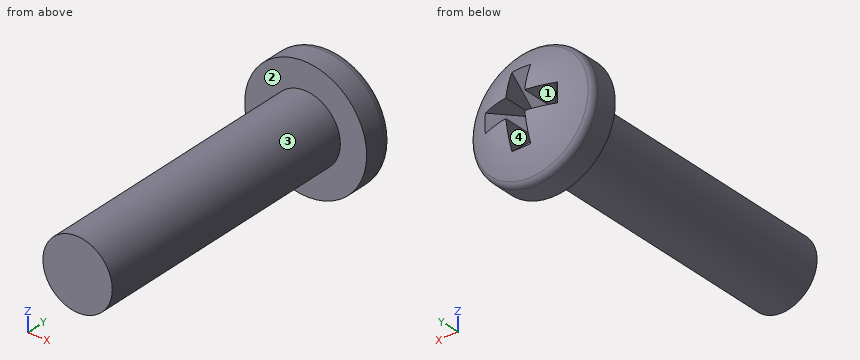
from build123d import *

# Parameters (mm, degrees)
SKETCH2_W          = 1.5875
SKETCH2_H          = 12.7
CUT_EXTRUDE1_DEPTH = 0.4318
CUT_EXTRUDE2_DEPTH = 0.4318


with BuildPart() as part:
    # Sketch1 → Base-Revolve (revolve)
    with BuildSketch(Plane.XY):
        with BuildLine():
            Line((0, 0), (2.794, 0))
            Line((2.794, 0), (2.794, 0.988051987))
            ThreePointArc((2.794, 0.988051987), (2.749892337, 1.170116122), (2.627350358, 1.311806977))
            ThreePointArc((2.627350358, 1.311806977), (1.379087386, 1.963971758), (0, 2.249624225))
            Line((0, 2.249624225), (0, 0))
        make_face()
    revolve(axis=Axis((0, 0, 0), (0, 1, 0)))

    # Sketch2 → Boss-Revolve1 (revolve)
    with BuildSketch(Plane.XY):
        with Locations((0.79375, -6.35)):
            Rectangle(SKETCH2_W, SKETCH2_H)
    revolve(axis=Axis((0, 0, 0), (0, 1, 0)))

    # Sketch3 → Cut-Extrude1 (cut, symmetric)
    with BuildSketch(Plane.XY):
        Polygon((-2.0193, 3.3909), (2.0193, 3.3909), (2.0193, 2.2606), (0, -0.0254), (-2.0193, 2.2606), align=None)
    extrude(amount=CUT_EXTRUDE1_DEPTH, both=True, mode=Mode.SUBTRACT)

    # Sketch4 → Cut-Extrude2 (cut, symmetric)
    with BuildSketch(Plane(origin=(0, 0, 0), x_dir=(0, 0, -1), z_dir=(1, 0, 0))):
        Polygon((-2.0193, 3.3909), (2.0193, 3.3909), (2.0193, 2.2606), (0, -0.0254), (-2.0193, 2.2606), align=None)
    extrude(amount=CUT_EXTRUDE2_DEPTH, both=True, mode=Mode.SUBTRACT)


solid = part.part
Check sheet for the modelled part. Datum: model origin and axes. Units: mm. Face numbers are marked on the shaded views. Coordinates: 2 decimals unless noted, no trailing zeros. Loops run counter-clockwise (first coordinate to the right, second up) from the corner with the lowest first, then second, coordinate; pieces in that order, holes last. Notation, with made-up numbers: (84.5, 53.5) -> (140.5, 53.5) arc R33 ccw to (140.5, 91.5) -> close; hole circle Ø1 at (24, 31.5). An arc over 180 degrees is marked (long way). Write item = value, one per line. Start each with the question number.
1. Section check B-B on y = -11. Record the cut outline in (x, z) (1 decimal), then the cut area to 3 significant figures.
2. Draft check along X on the marked faces 1, 2, 3 and 4. Enter one of: released by +X, released by -X, zero draft, split by the parting line, or undercut.
3. Section check A-A on y = 0.75. Record the cut outline in (x, z), then the cut area to 3 significant figures.
4. Material ranges on line 1 (Z direction, x = -0.1, y = -1.5); line 2 (Y direction, x = 0.4, z = 0.7); line 3 (Z direction, x = -0.4, y = -11.75), recorded low to high.
5. Depth check by flat-ended pin: P1, Ø1.3, axis at y = 1, z = 1, coming from the -X side; P2, Ø0.6, axis at y = 1.5, z = -1, coming from the -X side; P3, Ø1.3, axis at y = 1, z = -1, coming from the +X side. Enter the tip coordinate at first touch or a pass-through.
Responses:
q1.outline = circle Ø3.2 at (0, 0)
q1.area = 7.92 mm2
q2.face_1 = undercut
q2.face_2 = zero draft
q2.face_3 = split by the parting line
q2.face_4 = undercut
q3.outline = circle Ø5.59 at (0, 0); hole (-0.68, -0.43) -> (-0.43, -0.43) -> (-0.43, -0.68) -> (0.43, -0.68) -> (0.43, -0.43) -> (0.68, -0.43) -> (0.68, 0.43) -> (0.43, 0.43) -> (0.43, 0.68) -> (-0.43, 0.68) -> (-0.43, 0.43) -> (-0.68, 0.43) -> close
q3.area = 22.9 mm2
q4.line_1 = -1.58 to 1.58
q4.line_2 = -12.7 to 0.77
q4.line_3 = -1.54 to 1.54
q5.P1 = -2.77
q5.P2 = -2.57
q5.P3 = 2.77
